The listing builds one solid part. Answer for the finished solid, in the listing's coordinates (mm). A direction names the side the tool comes from. Round coordinates to 2 decimals unless told otherwise and drop trailing zeros. Loops run counter-clockwise (first coordinate to the right, second up) from the corner with the lowest first, then second, coordinate; pieces in that order, holes last. Notation, with made-up numbers: (-33.75, 22.25) - (-25.75, 22.25) arc R6 cw to (-25.75, 26.25) - close; hole circle Ø5 at (53, -6.75). An arc over 180 degrees is marked (long way). One line per question, with ' | ' between items. Start each with the question number.
Autodesk Fusion 360 part; units mm, degrees
sketch "Constraints Demo" plane through (0, 0, 0) normal (0, 1, 0) x (1, 0, 0)
  line L0 (41.0664, 18.1324) -> (104.0349, 18.1324)
  line L1 (104.0349, 18.1324) -> (104.0349, -34.6359)
  line L2 (104.0349, -34.6359) -> (130.6094, -34.6359)
  line L3 (130.6094, -34.6359) -> (130.6094, 18.1324)
  line L4 (130.6094, 18.1324) -> (193.5779, 18.1324)
  line L5 (193.5779, 18.1324) -> (193.5779, -78.8329)
  line L6 (193.5779, -78.8329) -> (134.7794, -86.972)
  line L7 (134.7794, -86.972) -> (99.8649, -86.972)
  line L8 (99.8649, -86.972) -> (83.789, -104.2824)
  line L9 (41.0664, 18.1324) -> (41.0664, -87.5042)
  arc A0 (41.0664, -87.5042) -> (83.789, -104.2824) centre (65.7223, -87.5042) ccw
  circle A1 centre (65.7223, -87.5042) radius 12.3567
  line L10 (117.3222, -86.972) -> (117.3222, -34.6359)
  line L11 (250, -100) -> (250, -35)
  spline S0 degree 5 poles (250, -35) (250, -32.6028) (250, -27.8084) (250.0776, -20.8345) (250.5826, -12.5726) (252.2639, -4.5288) (255.2107, 1.2852) (259.5207, 5.2526) (265.2004, 7.8511) (272.1693, 9.4403) (280.3152, 10.2655) (287.6902, 10.4323) (293.6726, 10.3106) (297.858, 10.1215) (300, 10) knots 0 0 0 0 0 0 0.1 0.2 0.3 0.4 0.5 0.6 0.7 0.8 0.9 1 1 1 1 1 1
  point P0 (260, 5)
extrude "Extrude1" add sketch "Constraints Demo" along normal blind 10
(1) Determine the mould class of faces 3 (the flat face through (117, 5, 34.636)), 4 (the flat face through (164.59, 4.93, 82.845)), 5 (the cylindrical face through (77.137, 4.93, 82.772)), 6 (the flat face through (118, 5, 86.972)) for opening direction X: pulls with the +X half, pulls with the -X half, needs draft (parallel to the pull), parting line crosses it, or undercut.
(2) Find section B-B on y = 1.5. Write down the section's boundary in (x, z), plus the area to 3 significant figures.
(3) A tool of negligible diameter and unlimited length cuts with its end or side. For faces 1 (the flat face through (116, 0, 46)), 2 (the flat face through (130.609, 5, 9)), from which of +Z, -Z, +X, -X, +Y, -Y can it reach the whole face along a straight path? Write none if from no direction.
(4) Find section C-C on x = 62. Write down the section's boundary in (y, z).
(5) Each of these flat-tipped pins is pushed along its axis until it touches: P1, Ø3, axis at x = 120, y = 3.5, coming from the +Z side; P2, Ø1.5, axis at x = 61, y = 8.5, coming from the +Z side; P3, Ø6, axis at x = 164, y = 8.5, coming from the +Z side; P4, Ø15, axis at x = 65.72, z = 87.5, coming from the +Y side. Where does it stop, or does it pass through?
(6) Find section D-D on x = 128. Write down the section's boundary in (y, z), plus the area to 3 significant figures.
(7) Consider L1, parallel to X at y = 1.5, z = 24; L2, parallel to Z at x = 65, y = 8.75; L3, parallel to Z at x = 104, y = 3.5. Determine where each line is inside the solid, lowest interval first.
(8) Find section A-A on z = 10. Write down the section's boundary in (x, y), plus the area to 3 significant figures.
Answer below:
1) face 3: undercut | face 4: pulls with the +X half | face 5: undercut | face 6: needs draft
2) outline: (41.07, -18.13) - (104.03, -18.13) - (104.03, 34.64) - (130.61, 34.64) - (130.61, -18.13) - (193.58, -18.13) - (193.58, 78.83) - (134.78, 86.97) - (99.86, 86.97) - (83.79, 104.28) arc R24.66 ccw to (41.07, 87.5) - close; hole circle Ø24.71 at (65.72, 87.5) | area: 14,900 mm2
3) face 1: +Z, -Z, +X, -X, -Y | face 2: -Z, +Y, -Y
4) outline: (0, -18.13) - (10, -18.13) - (10, 75.72) - (0, 75.72) - close; (0, 99.29) - (10, 99.29) - (10, 111.88) - (0, 111.88) - close
5) P1: z = 86.97 | P2: z = 111.84 | P3: z = 83.34 | P4: through
6) outline: (0, 34.64) - (10, 34.64) - (10, 86.97) - (0, 86.97) - close | area: 523 mm2
7) L1: 41.07 to 104.03, 130.61 to 193.58 | L2: -18.13 to 75.17, 99.84 to 112.15 | L3: -18.13 to 86.97
8) outline: (41.07, 0) - (104.03, 0) - (104.03, 10) - (41.07, 10) - close; (130.61, 0) - (193.58, 0) - (193.58, 10) - (130.61, 10) - close | area: 1,260 mm2
